The listing builds one solid part. Answer for the finished solid, in the listing's coordinates (mm). Give positions to 0.01 mm unless a question says otherwise; leave off trailing zeros. Order: outer loops, then holes, each group sorted by start corner. A loop starts at its lowest first (then second) coordinate and runs counter-clockwise, first axis right, second up. Notation, with made-up numbers: (37.5, 33) - (49.5, 33) arc R27 cw to (49.5, 66) - close; hole circle Ø8 at (67.25, 63.5). An arc over 180 degrees is marked (long way). Write each question's results on one line, items separated by ' | '. Start each with the question number.
1. Flat-ended cylindrical pins translate along their axes: pin 1 (1 mm diameter, centred on y = 1, z = -1.5, fed in from +X); pin 2 (0.8 mm diameter, centred on x = -32.5, z = -2, fed in from -Y); pin 3 (2 mm diameter, centred on y = 4.5, z = 1.5, fed in from +X); pin 4 (2 mm diameter, centred on x = -17, z = -2.5, fed in from +Y). Find the tip coordinate at first contact, or state that the pin passes through.
2. Section A-A (z = -3) is taken. Give the vertices of the cut face in (x, y).
3. Find the intervals of material crossed by L1, parallel to Y at x = -31.5, z = -1.75; L2, parallel to Z at x = -53.5, y = 3.5; L3, parallel to X at y = 1.25, z = -2.5, in increasing order.
4. Section D-D (y = 7.25) is taken. Give the vertices of the cut face in (x, z).
5. Section C-C (x = -46) is taken. Give the vertices of the cut face in (y, z), and give its area (3 significant figures).
from build123d import *

# Parameters (mm, degrees)
BOSS_EXTRUDE1_DEPTH = 2.5
CUT_EXTRUDE3_DEPTH  = 2.5
BOSS_EXTRUDE2_START = 3.8
BOSS_EXTRUDE2_DEPTH = 3.8
VARFILLET1_START    = -1
VARFILLET1_DEPTH    = 4


with BuildPart() as part:
    # Sketch1 → Boss-Extrude1 (new body)
    with BuildSketch(Plane.XY):
        with BuildLine():
            Line((-32.5, 0), (-32.5, 12))
            ThreePointArc((-32.5, 12), (-49.943474204, 9.23232597), (-65, 0))
            Line((-65, 0), (-34.616983549, 0))
            ThreePointArc((-34.616983549, 0), (-33.558491775, 0.00446614), (-32.5, 0))
        make_face()
        with BuildLine():
            Line((-30.383016451, 0), (0, 0))
            ThreePointArc((0, 0), (-15.056525796, 9.23232597), (-32.5, 12))
            Line((-32.5, 12), (-32.5, 0))
            ThreePointArc((-32.5, 0), (-31.441508225, 0.00446614), (-30.383016451, 0))
        make_face()
        with BuildLine():
            Line((0, -4), (0, 0))
            Line((0, 0), (-30.383016451, 0))
            ThreePointArc((-30.383016451, 0), (-15.068893895, -1.068651698), (0, -4))
        make_face()
        with BuildLine():
            Line((-34.616983549, 0), (-65, 0))
            Line((-65, 0), (-65, -4))
            ThreePointArc((-65, -4), (-49.931106105, -1.068651698), (-34.616983549, 0))
        make_face()
    extrude(amount=BOSS_EXTRUDE1_DEPTH)

    # Sketch2 → Cut-Extrude3 (cut)
    with BuildSketch(Plane.XY.offset(2.5)):
        with BuildLine():
            Line((-39, 2.5), (-32.5, 2.5))
            Line((-32.5, 2.5), (-32.5, 6))
            ThreePointArc((-32.5, 6), (-35.754530479, 5.860754323), (-39, 5.58095871))
            Line((-39, 5.58095871), (-39, 2.5))
        make_face()
        with BuildLine():
            ThreePointArc((-39, 5.58095871), (-35.754530479, 5.860754323), (-32.5, 6))
            Line((-32.5, 6), (-32.5, 6.5))
            Line((-32.5, 6.5), (-39, 6.5))
            Line((-39, 6.5), (-39, 5.58095871))
        make_face()
        with BuildLine():
            Line((-32.5, 6.5), (-32.5, 6))
            ThreePointArc((-32.5, 6), (-29.245469521, 5.860754323), (-26, 5.58095871))
            Line((-26, 5.58095871), (-26, 6.5))
            Line((-26, 6.5), (-32.5, 6.5))
        make_face()
        with BuildLine():
            Line((-32.5, 6), (-32.5, 2.5))
            Line((-32.5, 2.5), (-26, 2.5))
            Line((-26, 2.5), (-26, 5.58095871))
            ThreePointArc((-26, 5.58095871), (-29.245469521, 5.860754323), (-32.5, 6))
        make_face()
    extrude(amount=-CUT_EXTRUDE3_DEPTH, mode=Mode.SUBTRACT)

    # Sketch3 → Boss-Extrude2 (add)
    with BuildSketch(Plane(origin=(0, 0, 0), x_dir=(-1, 0, 0), z_dir=(0, 0, -1)).offset(BOSS_EXTRUDE2_START)):
        with BuildLine():
            Line((32.5, 10), (32.5, 12))
            ThreePointArc((32.5, 12), (31.800127405, 12.021886063), (31.1, 12.032943433))
            Line((31.1, 12.032943433), (31.1, 10))
            Line((31.1, 10), (32.5, 10))
        make_face()
        with BuildLine():
            ThreePointArc((33.9, 12.032943433), (33.199872595, 12.021886063), (32.5, 12))
            Line((32.5, 12), (32.5, 10))
            Line((32.5, 10), (33.9, 10))
            Line((33.9, 10), (33.9, 12.032943433))
        make_face()
        with BuildLine():
            ThreePointArc((31.1, 0.015701129), (31.800023358, 0.009933302), (32.5, 0))
            Line((32.5, 0), (32.5, 2.005619302))
            Line((32.5, 2.005619302), (31.1, 2.005619302))
            Line((31.1, 2.005619302), (31.1, 0.015701129))
        make_face()
        with BuildLine():
            Line((32.5, 2.005619302), (32.5, 0))
            ThreePointArc((32.5, 0), (33.199976642, 0.009933302), (33.9, 0.015701129))
            Line((33.9, 0.015701129), (33.9, 2.005619302))
            Line((33.9, 2.005619302), (32.5, 2.005619302))
        make_face()
    extrude(amount=-BOSS_EXTRUDE2_DEPTH)

    # VarFillet1: read off the stored shape, not the designer's step
    # VarFillet1 outline → VarFillet1 (cut)
    with BuildSketch(Plane.XY.offset(VARFILLET1_START)):
        with BuildLine():
            Line((0, -4), (0, -1.443114892))
            add(Edge.make_bspline(
                [(0, -1.443114892), (0, -3.973635887), (-2.462061436, -3.389007805)],
                knots=[0, 0, 0, 1, 1, 1], degree=2, weights=[1, 0.620068255, 1]))
            ThreePointArc((-2.462061436, -3.389007805), (-1.22948613, -3.688279812), (0, -4))
        make_face()
        with BuildLine():
            add(Edge.make_bspline(
                [(-0.671673321, 0.608863904), (0, 0.012143385), (0, -0.88631108)],
                knots=[0, 0, 0, 1, 1, 1], degree=2, weights=[1, 0.912185107, 1]))
            Line((0, -0.88631108), (0, 0))
            ThreePointArc((0, 0), (-0.334312348, 0.30611351), (-0.671673321, 0.608863904))
        make_face()
        with BuildLine():
            ThreePointArc((-65, -4), (-63.77051387, -3.688279812), (-62.537938564, -3.389007805))
            add(Edge.make_bspline(
                [(-62.537938564, -3.389007805), (-65, -3.973635887), (-65, -1.443114892)],
                knots=[0, 0, 0, 1, 1, 1], degree=2, weights=[1, 0.620068255, 1]))
            Line((-65, -1.443114892), (-65, -4))
        make_face()
        with BuildLine():
            add(Edge.make_bspline(
                [(-65, -0.88631108), (-65, 0.012143385), (-64.328326679, 0.608863904)],
                knots=[0, 0, 0, 1, 1, 1], degree=2, weights=[1, 0.912185107, 1]))
            ThreePointArc((-64.328326679, 0.608863904), (-64.665687652, 0.30611351), (-65, 0))
            Line((-65, 0), (-65, -0.88631108))
        make_face()
    extrude(amount=VARFILLET1_DEPTH, mode=Mode.SUBTRACT)


solid = part.part
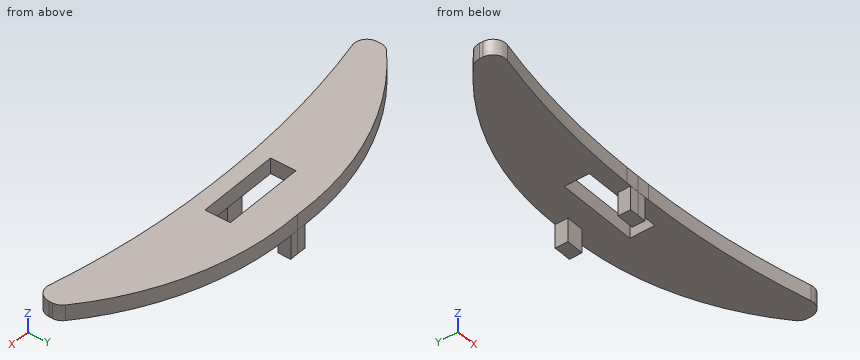
Reported:
1) pin 1: x = -31.1 | pin 2: y = 0 | pin 3: x = -4.28 | pin 4: through
2) outline: (-33.9, 0.02) arc R117.64 cw to (-32.5, 0) arc R117.64 cw to (-31.1, 0.02) - (-31.1, 2.01) - (-33.9, 2.01) - close; (-33.9, 10) - (-31.1, 10) - (-31.1, 12.03) arc R45.27 ccw to (-32.5, 12) arc R45.27 ccw to (-33.9, 12.03) - close
3) L1: 0.01 to 2.01, 10 to 12.03 | L2: 0 to 2.5 | L3: -33.9 to -31.1
4) outline: (-54.52, 0) - (-10.48, 0) - (-10.48, 2.5) - (-54.52, 2.5) - close
5) outline: (-0.61, 0) - (10.49, 0) - (10.49, 2.5) - (-0.61, 2.5) - close | area: 27.8 mm²
